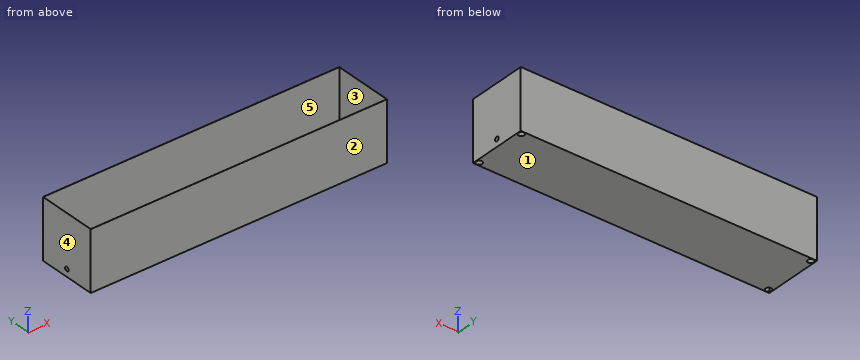
```python
from build123d import *

# Parameters (mm, degrees)
F0_W     = 2000
F0_H     = 400
F1_DEPTH = 400
F2_T     = -1
F5_D     = 40
F8_D     = 30


# Not quite as in the source:
# - the program builds the solid bodies; features that only make, move or delete a surface that nothing else refers to are left out


with BuildPart() as f1:
    # F0 (on Top) → F1 (new body)
    with BuildSketch(Plane.XY):
        Rectangle(F0_W, F0_H)
    extrude(amount=F1_DEPTH)

    # F2
    f2_openings = [f1.faces().sort_by_distance(p)[0] for p in [
        (0, 0, 400),
    ]]
    offset(amount=F2_T, openings=f2_openings)

    # F5 (through all)
    with Locations(Plane.XY.offset(1)):
        with Locations((977, 177), (977, -177), (-977, 177), (-977, -177)):
            Hole(F5_D / 2)

    # F8 (through all)
    with Locations(Plane(origin=(-1000, 0, 0), x_dir=(0, -1, 0), z_dir=(-1, 0, 0))):
        with Locations((0, 50)):
            Hole(F8_D / 2)


solid = f1.part
```
Geometry check sheet. Reference: the model listing, model coordinates, mm. Face numbers are marked on the shaded views. A direction names the side the tool comes from. Coordinates: 2 decimals unless noted, no trailing zeros. Order: outer loops, then holes, each group sorted by start corner. A loop starts at its lowest first (then second) coordinate and runs counter-clockwise, first axis right, second up.
Item 1: Mould release check, pull along Y, two halves, no side actions. Record for the marked faces 1, 2 and 3: released by +Y, released by -Y, zero draft, split by the parting line, or undercut.
Item 2: Section check A-A (x = -977). Enter the section's corners in (y, z).
Item 3: Section check B-B (z = 365.5). Enter the section's corners in (x, y), plus the area to 3 significant figures.
Item 4: Section check D-D (y = 112). Enter the section's corners in (x, z).
Item 5: Scan lines: line 1 along Y through (x, z) = (977, 0.3); line 2 along Y through (x, z) = (-817.5, 144); line 3 along Z through (x, y) = (999.8, 0). Record each from-to range of solid material in increasing order.
Item 6: Section check C-C (x = -202). Enter the section's corners in (y, z).
Item 7: Tool access check on the marked faces 4 and 5. Record the directions out of +Z, -Z, +X, -X, +Y, -Y that give a thin tool (end or side, any length) a straight path to the whole face; none if there is none.
Item 8: Depth check by flat-ended pin: pin 1 (24 mm diameter, centred on y = 0, z = 50, fed in from -X); pin 2 (3 mm diameter, centred on x = 538, y = 10, fed in from +Z); pin 3 (6 mm diameter, centred on x = 393, y = 78, fed in from -Z). Enter the tip coordinate at first touch or a pass-through.
Check sheet entries:
1. face 1: zero draft
1. face 2: released by -Y
1. face 3: undercut
2. outline: (-200, 0) - (-197, 0) - (-197, 1) - (-199, 1) - (-199, 400) - (-200, 400) - close; (-157, 0) - (157, 0) - (157, 1) - (-157, 1) - close; (197, 0) - (200, 0) - (200, 400) - (199, 400) - (199, 1) - (197, 1) - close
3. outline: (-1000, -200) - (1000, -200) - (1000, 200) - (-1000, 200) - close; hole (-999, -199) - (999, -199) - (999, 199) - (-999, 199) - close
3. area: 4,800 mm2
4. outline: (-1000, 0) - (1000, 0) - (1000, 400) - (999, 400) - (999, 1) - (-999, 1) - (-999, 400) - (-1000, 400) - close
5. line 1: y = -200 to -197, -157 to 157, 197 to 200
5. line 2: y = -200 to -199, 199 to 200
5. line 3: z = 0 to 35, 65 to 400
6. outline: (-200, 0) - (200, 0) - (200, 400) - (199, 400) - (199, 1) - (-199, 1) - (-199, 400) - (-200, 400) - close
7. face 4: +Z, -Z, -X, +Y, -Y
7. face 5: +Z
8. pin 1: passes through
8. pin 2: stops at z = 1
8. pin 3: stops at z = 0
